```python
from build123d import *

# Parameters (mm, degrees)
BOSS_EXTRUDE1_DEPTH = 0.79375
BOSS_EXTRUDE2_DEPTH = 482.6
SKETCH5_W           = 30.221142114
SKETCH5_H           = 4.701476641
CUT_EXTRUDE1_DEPTH  = 27.94


with BuildPart() as part:
    # Sketch1 → Boss-Extrude1 (new body)
    with BuildSketch(Plane(origin=(-94.488, 0, 0), x_dir=(0, -1, 0), z_dir=(-1, 0, 0))):
        Polygon((111.125, -196.85), (111.125, -203.2), (85.725, -203.2), (85.725, -196.85), (60.325, -196.85), (60.325, -682.625), (85.725, -682.625), (85.725, -679.45), (111.125, -679.45), (111.125, -682.625), (136.525, -682.625), (136.525, -290.406498707), (136.525, -203.2), (136.525, -196.85), align=None)
        with BuildLine():
            Line((149.225, -203.2), (136.525, -203.2))
            Line((136.525, -203.2), (136.525, -290.406498707))
            ThreePointArc((136.525, -290.406498707), (137.30121982, -286.034603668), (139.534994681, -282.197126202))
            Line((139.534994681, -282.197126202), (184.118202659, -229.57294303))
            ThreePointArc((184.118202659, -229.57294303), (185.23509009, -227.654204297), (185.6232, -225.468256778))
            Line((185.6232, -225.468256778), (185.6232, -203.2))
            Line((185.6232, -203.2), (168.275, -203.2))
            Line((168.275, -203.2), (168.275, -196.85))
            Line((168.275, -196.85), (149.225, -196.85))
            Line((149.225, -196.85), (149.225, -203.2))
        make_face()
    extrude(amount=-BOSS_EXTRUDE1_DEPTH)

    # Sketch4 → Boss-Extrude2 (add)
    with BuildSketch(Plane(origin=(0, 0, -679.45), x_dir=(-1, 0, 0), z_dir=(0, 0, -1))):
        with BuildLine():
            Line((97.166105032, -116.822884411), (94.488, -136.525))
            Line((94.488, -136.525), (94.488, -114.25313135))
            Line((94.488, -114.25313135), (94.488, -111.125))
            Line((94.488, -111.125), (94.488, -108.585))
            ThreePointArc((94.488, -108.585), (95.231948776, -110.381051224), (97.028, -111.125))
            Line((97.028, -111.125), (113.793536469, -111.125))
            ThreePointArc((113.793536469, -111.125), (114.50064325, -111.417893219), (114.793536469, -112.125))
            Line((114.793536469, -112.125), (114.793536469, -113.625))
            ThreePointArc((114.793536469, -113.625), (114.50064325, -114.332106781), (113.793536469, -114.625))
            Line((113.793536469, -114.625), (99.682959601, -114.625))
            ThreePointArc((99.682959601, -114.625), (98.012237242, -115.251812399), (97.166105032, -116.822884411))
        make_face()
    extrude(amount=-BOSS_EXTRUDE2_DEPTH)

    # Sketch5 → Cut-Extrude1 (cut)
    with BuildSketch(Plane(origin=(-93.69425, 0, 0), x_dir=(0, 0, -1), z_dir=(1, 0, 0))):
        with Locations((188.089428943, -108.77426168)):
            Rectangle(SKETCH5_W, SKETCH5_H)
    extrude(amount=-CUT_EXTRUDE1_DEPTH, mode=Mode.SUBTRACT)


solid = part.part
```
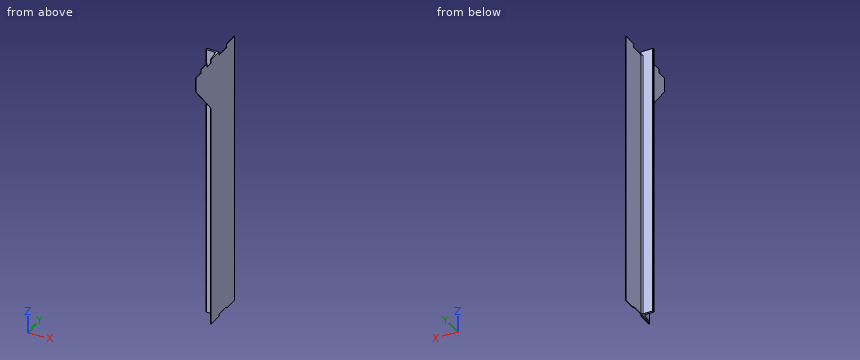
Input: part model. Units: mm. Frame: model coordinates. Coordinates: 2 decimals unless noted, no trailing zeros. Write each loop counter-clockwise with the first axis right and the second up, starting at its lowest first coordinate (ties: lowest second). Pieces come first, ordered by that corner, then holes. Notation, with made-up numbers: M -3,21.25 L 34,21.25 A30 cw 34,51.25 Z; hole C 62,7.5 d3. An arc over 180 degrees is marked long. Use one line per item in the form item = value.
Q1. Material intervals for probe 1 along Y at (x, z) = (-102.75, -243) (3 decimals); probe 2 along X at (y, z) = (-118.5, -630); probe 3 along X at (y, z) = (-105.5, -627.5), sorted ascending. Write a range as from..to.
Answer below:
probe_1 = -114.625..-111.125
probe_2 = -96.94..-93.69
probe_3 = -94.49..-93.69
Q2. Section A-A (z = -434.5). Return loops of the section in (x, y) (3 decimals), plus the area to 3 significant figures.
Answer below:
outline = M -114.794,-113.625 A1 ccw -113.794,-114.625 L -99.683,-114.625 A2.54 cw -97.166,-116.823 L -94.488,-136.525 L -93.694,-136.525 L -93.694,-60.325 L -94.488,-60.325 L -94.488,-108.585 A2.54 cw -97.028,-111.125 L -113.794,-111.125 A1 ccw -114.794,-112.125 Z
area = 166 mm²
Q3. Section C-C (y = -176.5). Return loops of the section in (x, z).
Answer below:
outline = M -94.49,-238.57 L -93.69,-238.57 L -93.69,-203.2 L -94.49,-203.2 Z
Q4. Section B-B (x = -105). Return loops of the section in (y, z) (3 decimals).
Answer below:
outline = M -114.625,-679.45 L -111.125,-679.45 L -111.125,-196.85 L -114.625,-196.85 Z
Q5. Section D-D (z = -255). Return loops of the section in (x, y) (3 decimals).
Answer below:
outline = M -114.794,-113.625 A1 ccw -113.794,-114.625 L -99.683,-114.625 A2.54 cw -97.166,-116.823 L -94.488,-136.525 L -94.488,-162.576 L -93.694,-162.576 L -93.694,-60.325 L -94.488,-60.325 L -94.488,-108.585 A2.54 cw -97.028,-111.125 L -113.794,-111.125 A1 ccw -114.794,-112.125 Z
Q6. First-contact query: pin 1 (1 mm diameter, centred on y = -111, z = -608.5, fed in from -X); pin 2 (24.5 mm diameter, centred on y = -158, z = -262.5, fed in from -X); pin 3 (3.5 mm diameter, centred on x = -95, y = -101, fed in from +Z); pin 4 (6 mm diameter, centred on x = -98, y = -171, fed in from -Z). Flat tips, straight axial feed; report the tip coordinate or a pass-through.
Answer below:
pin_1 = -114.57
pin_2 = -94.49
pin_3 = -203.2
pin_4 = through
